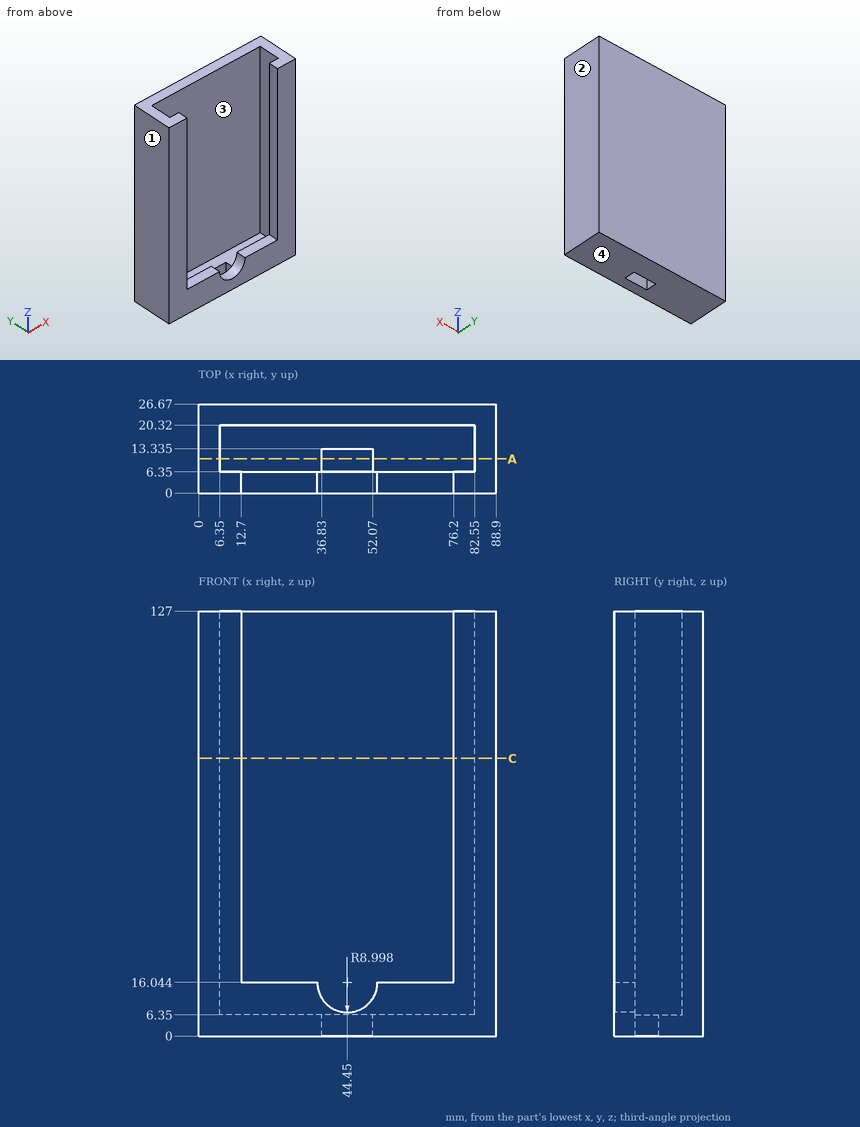
Source: three-view drawing plus pictorial views. Frame: mm from the lowest corner of the part. Give positions to 0.01 mm unless a question says otherwise; leave off trailing zeros. Order: outer loops, then holes, each group sorted by start corner. A loop starts at its lowest first (then second) coordinate and runs counter-clockwise, first axis right, second up. Notation, with made-up numbers: (0, 18) -> (56, 18) arc R27 ccw to (56, 47) -> close; hole circle Ø1 at (-16, -22.5). An arc over 180 degrees is marked (long way). Write each question's results on one line, items separated by ' | '. Start each with the question number.
Item 1: Cut plane A-A on y = 10.25. Return the cut outline in (x, z), then the cut area to 3 significant figures.
Item 2: Contact query for flat-ended pins moving along their axis: P1, Ø8, axis at y = 4.5, z = 29, coming from the -X side; P2, Ø5, axis at x = 61.5, y = 4, coming from the +Z side; P3, Ø12, axis at x = 26.5, z = 49.5, coming from the -Y side; P4, Ø7, axis at x = 35.5, y = 14.5, coming from the +Z side. Output: stop coordinate, or through.
Item 3: Line query: line 1 (X direction, y = 3.5, z = 30.5); line 2 (X direction, y = 15, z = 81); line 3 (Y direction, x = 16, z = 14.5). Output: solid intervals per line, ascending.
Item 4: Mould query, pull axis X, two halves, no side actions, for the marked faces 1, 2, 3 and 4. Classes: pulls with the +X half, pulls with the -X half, needs draft (parallel to the pull), parting line crosses it, or undercut.
Item 5: Cut plane C-C on z = 83. Return the cut outline in (x, y), then the cut area to 3 significant figures.
Established:
1) outline: (0, 0) -> (36.83, 0) -> (36.83, 6.35) -> (6.35, 6.35) -> (6.35, 127) -> (0, 127) -> close; (52.07, 0) -> (88.9, 0) -> (88.9, 127) -> (82.55, 127) -> (82.55, 6.35) -> (52.07, 6.35) -> close | area: 2,000 mm^2
2) P1: x = 0 | P2: z = 16.04 | P3: y = 20.32 | P4: z = 6.35
3) line 1: 0 to 12.7, 76.2 to 88.9 | line 2: 0 to 6.35, 82.55 to 88.9 | line 3: 0 to 6.35, 20.32 to 26.67
4) face 1: pulls with the -X half | face 2: pulls with the +X half | face 3: undercut | face 4: needs draft
5) outline: (0, 0) -> (12.7, 0) -> (12.7, 6.35) -> (6.35, 6.35) -> (6.35, 20.32) -> (82.55, 20.32) -> (82.55, 6.35) -> (76.2, 6.35) -> (76.2, 0) -> (88.9, 0) -> (88.9, 26.67) -> (0, 26.67) -> close | area: 903 mm^2
